Autodesk Inventor part; units mm, degrees
ref_plane "YZ Plane" through (0, 0, 0) normal (1, 0, 0) x (0, 1, 0)
ref_plane "XZ Plane" through (0, 0, 0) normal (0, 1, 0) x (-1, 0, 0)
ref_plane "XY Plane" through (0, 0, 0) normal (0, 0, 1) x (1, 0, 0)
sketch "スケッチ1" plane through (0, 0, 0) normal (0, 1, 0) x (-1, 0, 0)
  line L0 (20, -20) -> (-20, -20)
  line L1 (-20, -20) -> (-20, 20)
  line L2 (-20, 20) -> (20, 20)
  line L3 (20, 20) -> (20, -20)
  line L4 (-20, 20) -> (20, -20) construction
  line L5 (-20, -20) -> (20, 20) construction
  point P0 (0, 0)
  point P1 (0, 0)
  dimension "d0" = 40
  dimension "d1" = 40
extrude "押し出し1" add sketch "スケッチ1" along normal blind 3
sketch "スケッチ2" plane through (0, 3, 0) normal (0, 1, 0) x (1, 0, 0)
  line L0 (-20, -20) -> (20, -20)
  line L1 (20, -20) -> (20, 20)
  line L2 (20, 20) -> (-20, 20)
  line L3 (-20, 20) -> (-20, -20)
  line L4 (-20, -20) -> (20, -20)
  line L5 (-20, -20) -> (-17, -20)
  line L6 (-17, -20) -> (-17, 20)
  line L7 (-17, 20) -> (-20, 20)
  line L8 (-20, 20) -> (-20, -20)
  line L9 (20, -20) -> (20, 20)
  line L10 (20, -20) -> (17, -20)
  line L11 (17, -20) -> (17, 20)
  line L12 (17, 20) -> (20, 20)
  line L13 (20, 20) -> (20, -20)
  line L14 (20, 20) -> (-20, 20)
  point P0 (0, 0)
  point P1 (-17, 20)
  dimension "d4" = 3
  dimension "d5" = 3
extrude "押し出し2" add sketch "スケッチ2" along normal blind 40 from surface at -3 contours L3 L2 L6 L0 | L11 L2 L1 L0
sketch "スケッチ3" plane through (20, 0, 20) normal (1, 0, 0) x (0, 0, -1)
  line L0 (0, 3) -> (40, 3)
  line L1 (25, 18) -> (40, 18) construction
  line L2 (40, 40) -> (40, 3) construction
  line L3 (25, 18) -> (-0.078171, 18) construction
  point P0 (20, 0)
  dimension "d8" = 15
  dimension "d50" = 15
hole "穴1" at (20, 18, -5) direction (-1, 0, 0) diameter 7 end through all
sketch "スケッチ5" plane through (20, 0, 20) normal (1, 0, 0) x (0, 0, -1)
  line L0 (0, 0) -> (0, 40)
  line L1 (0, 0) -> (40, 0)
  line L2 (36, 33) -> (6, 33)
  line L3 (6, 33) -> (6, 3)
  line L4 (6, 3) -> (36, 3)
  line L5 (36, 3) -> (36, 33)
  line L6 (36, 33) -> (6, 3) construction
  line L7 (36, 3) -> (6, 33) construction
  line L8 (36, 18) -> (6, 18)
  circle A0 centre (25, 18) radius 3.5
  point P0 (20, 0)
  point P1 (21, 18)
  point P2 (30, 27)
  point P3 (12, 27)
  point P4 (21, 18)
  point P5 (12, 9)
  point P6 (21, 18)
  point P7 (30, 9)
  point P8 (21, 18)
  point P9 (30, 27)
  dimension "d20" = 30
  dimension "d21" = 30
  dimension "d23" = 6
  dimension "d24" = 6
  dimension "d27" = 360
  dimension "d40" = 4
hole "穴2" at (20, 27, -10) at (20, 9, -10) at (20, 27, 8) at (20, 9, 8) direction (-1, 0, 0) diameter 2.459 depth 3
sketch "スケッチ6" plane through (0, 3, 0) normal (0, 1, 0) x (1, 0, 0)
  line L0 (17, 20) -> (-17, 20)
  point P0 (0, 0)
  point P1 (0, 15)
  point P2 (0, -5)
  point P3 (0, 20)
  dimension "d41" = 5
  dimension "d42" = 20
hole "穴3" at (0, 3, -15) at (0, 3, 5) direction (0, -1, 0) diameter 2.459 depth 3
sketch "スケッチ7" plane through (20, 0, 20) normal (1, 0, 0) x (0, 0, -1)
  circle A0 centre (25, 18) radius 3.5
  line L0 (25, 18) -> (-12.331112, 18)
  line L1 (-6.275173, 36.05673) -> (25, 18)
  circle A1 centre (5, 27.814955) radius 1.5
  line L2 (0, 0) -> (0, 40)
  point P0 (20, 0)
  dimension "d51" = 30
  dimension "d52" = 3
  dimension "d53" = 5
extrude "押し出し4" cut sketch "スケッチ7" against normal up to surface (40 mm away) contours A1
equation "\"d54\" = d53"
properties part number "hand" material "アルミニウム 6061"
Geometry check sheet. Reference: the model listing, model coordinates, mm. A direction names the side the tool comes from. Round coordinates to 2 decimals unless told otherwise and drop trailing zeros. Order: outer loops, then holes, each group sorted by start corner. A loop starts at its lowest first (then second) coordinate and runs counter-clockwise, first axis right, second up. Notation, with made-up numbers: M -30,42 L -17,42 A29 cw -17,77 Z; hole C -19.75,5 d4. An arc over 180 degrees is marked long. Answer as CSV lines item,"result".
1) Sectioned sample at D-D on z = 5. Record the cut outline in (x, y), and give its area (3 significant figures).
Entries:
outline,"M -20,0 L -1.23,0 L -1.23,3 L -17,3 L -17,40 L -20,40 Z; M 1.23,0 L 20,0 L 20,40 L 17,40 L 17,3 L 1.23,3 Z"
area,"335 mm2"
2) Sectioned sample at C-C on x = 0. Record the cut outline in (y, z).
Entries:
outline,"M 0,-20 L 3,-20 L 3,-16.23 L 0,-16.23 Z; M 0,-13.77 L 3,-13.77 L 3,3.77 L 0,3.77 Z; M 0,6.23 L 3,6.23 L 3,20 L 0,20 Z"
3) Thickness scan on probe 1 along Z at (x, y) = (0, 1); probe 2 along Y at (x, z) = (19.1, 8); probe 3 along Z at (x, y) = (17.7, 9). Record the ranges inside material, lowest first. Write a range as [from, to].
Entries:
probe 1,"[-20, -16.23], [-13.77, 3.77], [6.23, 20]"
probe 2,"[0, 7.77], [10.23, 25.77], [28.23, 40]"
probe 3,"[-20, -11.23], [-8.77, 6.77], [9.23, 20]"
4) Gauge pin test, flat ends, axial feed: pin 1 Ø2 at (x, z) = (0, -15) entering from +Y; pin 2 Ø1.5 at (y, z) = (27, 8) entering from +X; pin 3 Ø9 at (y, z) = (18, -5) entering from +X; pin 4 Ø3 at (x, z) = (11, -9) entering from +Y. Record the tip position at first contact, or that the pin passes through.
Entries:
pin 1,"through"
pin 2,"x = -17"
pin 3,"x = 20"
pin 4,"y = 3"
5) Sectioned sample at B-B on y = 11. Record the cut outline in (x, z), and give its area (3 significant figures).
Entries:
outline,"M -20,-20 L -17,-20 L -17,20 L -20,20 Z; M 17,-20 L 20,-20 L 20,20 L 17,20 Z"
area,"240 mm2"
6) Mould release check, pull along X, two halves, no side actions. Record for faces 1 (the face through (-20, 20, 0)), 2 (the face through (18.52, 26.35, 15.33)), 3 (the face through (-0.369, 1.479, -13.827)), 4 (the face through (0, 3, 0)): +X half, -X half, draft (parallel to the pull), parting line (faces both ways), or undercut.
Entries:
face 1,"-X half"
face 2,"draft"
face 3,"undercut"
face 4,"undercut"
7) Sectioned sample at A-A on z = -10. Record the cut outline in (x, y), and give its area (3 significant figures).
Entries:
outline,"M -20,0 L 20,0 L 20,7.77 L 17,7.77 L 17,3 L -17,3 L -17,40 L -20,40 Z; M 17,10.23 L 20,10.23 L 20,25.77 L 17,25.77 Z; M 17,28.23 L 20,28.23 L 20,40 L 17,40 Z"
area,"327 mm2"
8) Tool access check on faces 5 (the face through (18.48, 28.2, 8.27)), 6 (the face through (-17, 21, 0)), 7 (the face through (-18.48, 26.35, 15.33)). Record the directions out of +Z, -Z, +X, -X, +Y, -Y that give a thin tool (end or side, any length) a straight path to the whole face; none if there is none.
Entries:
face 5,"+X"
face 6,"+Z, -Z, +Y"
face 7,"+X, -X"
